from build123d import *

# Parameters (mm, degrees)
BOSS_EXTRUDE1_DEPTH = 127


with BuildPart() as part:
    # Sketch5 → Boss-Extrude1 (new body)
    with BuildSketch(Plane(origin=(0, 0, 0), x_dir=(1, 0, 0), z_dir=(0, 1, 0))):
        Polygon((-35.906793393, -108.580423135), (-28.596428271, -110.730530524), (3.655182561, -1.075053694), (-3.655182561, 1.075053694), align=None)
        Polygon((-3.010150344, -5.733619704), (-0.57336197, -6.450322166), (-29.241460488, -103.921857126), (-31.678248862, -103.205154663), align=None, mode=Mode.SUBTRACT)
    extrude(amount=-BOSS_EXTRUDE1_DEPTH)


solid = part.part
CAD build for the part. Positions are in the model's coordinates, mm. Coordinates: 2 decimals unless noted, no trailing zeros. Write each loop counter-clockwise with the first axis right and the second up, starting at its lowest first coordinate (ties: lowest second). Pieces come first, ordered by that corner, then holes. Notation, with made-up numbers: (-3, -6.75) - (55, -6.75) arc R19 ccw to (55, 11.25) - close; hole circle Ø10 at (10.25, 61). An arc over 180 degrees is marked (long way). Use a Markdown table: item, result. Add a question column.
Item 1: Mould opens along X. For faces 1 (the face through (-17.545, -62.611, 55.152)), 2 (the face through (-18, 0, 55)), 3 (the face through (-14.707, -62.611, 54.504)), 4 (the face through (-19.555, -62.611, 52.985)) say: pulls with the +X half, pulls with the -X half, needs draft (parallel to the pull), parting line crosses it, or undercut.
Item 2: Band-saw the part on D-D, the plane x = 1.5. Give the cut face in (y, z).
Item 3: Band-saw the part on C-C, the plane z = 63.5. Give the cut face in (x, y), and give its area (3 significant figures).
Item 4: Flat gauge pins, fed straight in: pin 1 (8 mm diameter, centred on y = -64, z = 80, fed in from +X); pin 2 (3 mm diameter, centred on x = -1, y = -21, fed in from -Z); pin 3 (5 mm diameter, centred on y = -98, z = 80.5, fed in from +X). Where does each tip first touch, or does it go through?
Item 5: Band-saw the part on A-A, the plane y = -37.5. Give the cut face in (x, z), and give its area (3 significant figures).
Item 6: Band-saw the part on B-B, the plane x = -8. Give the cut face in (y, z).
Item 7: Drill centre lines: L1, parallel to X at y = -108.5, z = 95.5; L2, parallel to X at y = -72.5, z = 74.5. Where is each one in solid material? Low to high. Write a range as from..to.
Numbers:
| question | item | result |
|---|---|---|
| 1 | face 1 | undercut |
| 1 | face 2 | needs draft |
| 1 | face 3 | undercut |
| 1 | face 4 | pulls with the -X half |
| 2 | outline | (-127, 0.44) - (0, 0.44) - (0, 8.4) - (-127, 8.4) - close |
| 3 | outline | (-22.65, -127) - (-20, -127) - (-20, 0) - (-22.65, 0) - close; (-17.35, -127) - (-14.71, -127) - (-14.71, 0) - (-17.35, 0) - close |
| 3 | area | 672 mm2 |
| 4 | pin 1 | x = -18.38 |
| 4 | pin 2 | z = -0.74 |
| 4 | pin 3 | x = -18.97 |
| 5 | outline | (-35.91, 108.58) - (-3.66, -1.08) - (3.66, 1.08) - (-28.6, 110.73) - close; hole (-31.68, 103.21) - (-3.01, 5.73) - (-0.57, 6.45) - (-29.24, 103.92) - close |
| 5 | area | 613 mm2 |
| 6 | outline | (-127, 13.7) - (0, 13.7) - (0, 22.7) - (-127, 22.7) - close; (-127, 31.7) - (0, 31.7) - (0, 40.7) - (-127, 40.7) - close |
| 7 | L1 | -32.06..-29.41, -26.76..-24.12 |
| 7 | L2 | -25.88..-23.24, -20.59..-17.94 |
